Check sheet for the drawn part. Datum: minimum x, y, z corner. Units: mm. Coordinates: 2 decimals unless noted, no trailing zeros. Write each loop counter-clockwise with the first axis right and the second up, starting at its lowest first coordinate (ties: lowest second). Pieces come first, ordered by that corner, then holes. Notation, with made-up numbers: (30.25, 14.5) -> (63.25, 14.5) arc R34 cw to (63.25, 48.5) -> close; hole circle Ø7 at (69.5, -8.5). An arc over 180 degrees is marked (long way). Answer in a Markdown table with one row per item. Add a question column.
Q1. Gauge pin test, flat ends, axial feed: P1, Ø0.5, axis at x = 24.5, y = 2.5, coming from the -Z side; P2, Ø4, axis at x = 18.5, z = 4.5, coming from the -Y side. Record the tip position at first contact, or that the pin passes through.
Q2. Thickness scan on line 1 (Z direction, x = 11.5, y = 2.3); line 2 (Y direction, x = 6.5, z = 8.75); line 3 (Z direction, x = 3, y = 2.45). Record the ranges inside material, lowest first.
Q3. Section check A-A, the plane y = 2.55. Record the boundary of the cut face in (x, z).
Q4. Section check B-B, the plane z = 6.25. Record the boundary of the cut face in (x, y).
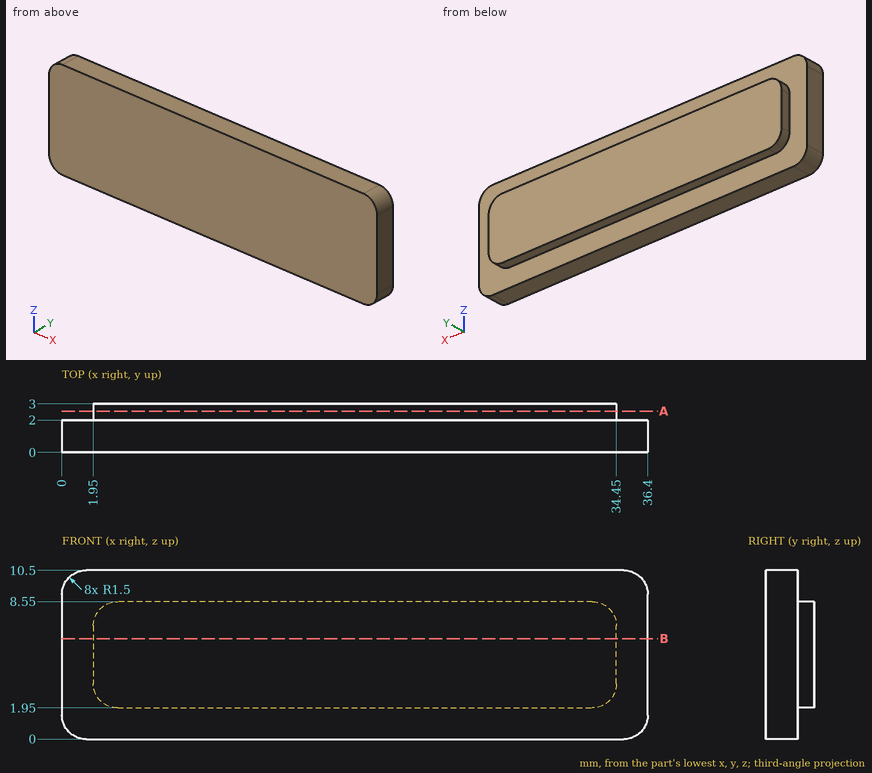
Calculated:
| question | item | result |
|---|---|---|
| 1 | P1 | stops at z = 1.95 |
| 1 | P2 | stops at y = 0 |
| 2 | line 1 | z = 1.95 to 8.55 |
| 2 | line 2 | y = 0 to 2 |
| 2 | line 3 | z = 2.02 to 8.48 |
| 3 | outline | (1.95, 3.45) arc R1.5 ccw to (3.45, 1.95) -> (32.95, 1.95) arc R1.5 ccw to (34.45, 3.45) -> (34.45, 7.05) arc R1.5 ccw to (32.95, 8.55) -> (3.45, 8.55) arc R1.5 ccw to (1.95, 7.05) -> close |
| 4 | outline | (0, 0) -> (36.4, 0) -> (36.4, 2) -> (34.45, 2) -> (34.45, 3) -> (1.95, 3) -> (1.95, 2) -> (0, 2) -> close |
